The listing builds one solid part. Answer for the finished solid, in the listing's coordinates (mm). Face numbers are marked on the shaded views. Coordinates: 2 decimals unless noted, no trailing zeros. Write each loop counter-clockwise with the first axis right and the second up, starting at its lowest first coordinate (ties: lowest second). Pieces come first, ordered by that corner, then holes. Notation, with made-up numbers: M 6,21.25 L 47,21.25 A27 cw 47,52.25 Z; hole C -2,66.25 d8. An arc over 180 degrees is marked long. Answer as CSV lines item,"result". Start each with the question number.
```python
from build123d import *

# Parameters (mm, degrees)
SKETCH1_W                            = 398.78
SKETCH1_H                            = 101.6
BOSS_EXTRUDE1_DEPTH                  = 3.81
SKETCH11_W                           = 100.33
SKETCH11_H                           = 25.4
CUT_EXTRUDE1_DEPTH                   = 206.794869227
F_5_16_0_3125_DIAMETER_HOLE1_D       = 7.9375
F_6_CLEARANCE_HOLE1_D                = 3.6576
F_8_CLEARANCE_HOLE1_D                = 4.4958
LPATTERN1_COUNT                      = 2
LPATTERN1_PITCH                      = 328.93
F_11_64_0_17188_DIAMETER_HOLE2_D     = 4.365752
F_11_64_0_17188_DIAMETER_HOLE2_DEPTH = 8.89
F_11_64_0_17188_DIAMETER_HOLE2_TIP   = 1.311604225


with BuildPart() as part:
    # Sketch1 → Boss-Extrude1 (new body)
    with BuildSketch(Plane.XY):
        Rectangle(SKETCH1_W, SKETCH1_H)
    extrude(amount=BOSS_EXTRUDE1_DEPTH)

    # Sketch11 → Cut-Extrude1 (cut, through all)
    with BuildSketch(Plane.XY.offset(3.81)):
        with Locations((-53.975, -38.1)):
            Rectangle(SKETCH11_W, SKETCH11_H)
    extrude(amount=-CUT_EXTRUDE1_DEPTH, mode=Mode.SUBTRACT)

    # 5/16 (0.3125) Diameter Hole1 (through all)
    with Locations(Plane.XY.offset(3.81)):
        with Locations((11.074908, -43.18)):
            Hole(F_5_16_0_3125_DIAMETER_HOLE1_D / 2)

    # #6 Clearance Hole1 (through all)
    with Locations(Plane.XY.offset(3.81)):
        with Locations((132.715, -15.24), (196.215, -16.51), (196.215, 12.7), (196.215, 38.1), (132.715, 45.72), (132.715, 15.24), (132.715, -45.72), (196.215, -45.72)):
            f_6_clearance_hole1 = Hole(F_6_CLEARANCE_HOLE1_D / 2)

    # #8 Clearance Hole1 (through all)
    with Locations(Plane.XY.offset(3.81)):
        with Locations((180.34, 44.45), (180.34, 19.05), (180.34, -6.35), (-116.84, 44.45), (-116.84, 19.05), (-116.84, -6.35)):
            Hole(F_8_CLEARANCE_HOLE1_D / 2)

    # LPattern1: #6 Clearance Hole1 ×2
    with Locations(*[(-i * LPATTERN1_PITCH, 0, 0) for i in range(1, LPATTERN1_COUNT)]):
        add(f_6_clearance_hole1, mode=Mode.SUBTRACT)

    # 11/64 (0.17188) Diameter Hole2
    with Locations(Plane.XY.offset(3.81)):
        with Locations((-5.715, 6.35), (6.985, 6.35)):
            Hole(F_11_64_0_17188_DIAMETER_HOLE2_D / 2, depth=F_11_64_0_17188_DIAMETER_HOLE2_DEPTH)
            with Locations((0, 0, -(F_11_64_0_17188_DIAMETER_HOLE2_DEPTH + F_11_64_0_17188_DIAMETER_HOLE2_TIP / 2))):  # 118° drill point
                Cone(0, F_11_64_0_17188_DIAMETER_HOLE2_D / 2, F_11_64_0_17188_DIAMETER_HOLE2_TIP, mode=Mode.SUBTRACT)


solid = part.part
```
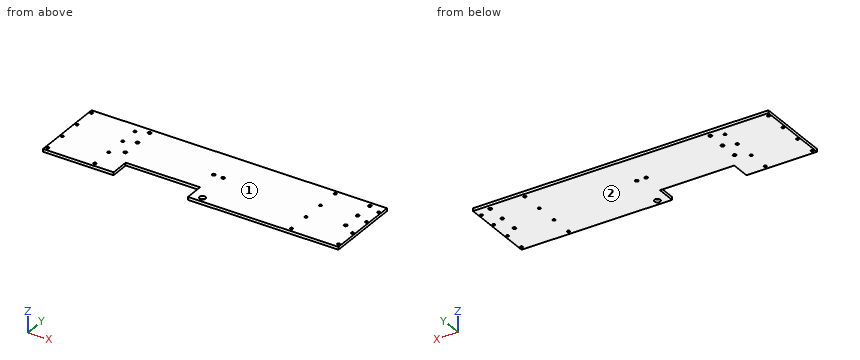
1) The part is cut by section C-C (x = -49). Determine the outline of the cut face in (y, z), then the cut area to 3 significant figures.
2) For a pull along Z with two mould halves and no side action, classify the marked faces 1 and 2 as +Z half, -Z half, draft (parallel to the pull), parting line (faces both ways), or undercut.
3) The part is cut by section A-A (y = -30). Determine the outline of the cut face in (x, z).
4) This flat-tipped pin is pushed along its axis until it touches: P1, Ø2, axis at x = 196.215, y = 12.7, coming from the -Z side. Where does it stop, or does it pass through?
5) Find the intervals of material crossed by line 1 (X direction, y = 18.5, z = 1.25); line 2 (X direction, y = -26, z = 3.3); line 3 (X direction, y = 14, z = 3.45), in increasing order. Write a range as from..to.
6) The part is cut by section B-B (z = 1.8). Count the separate pieces of the cut face and the enclosed holes in it, then the cut area to 3 significant figures.
Completed:
1,outline,"M -25.4,0 L 50.8,0 L 50.8,3.81 L -25.4,3.81 Z"
1,area,"290 mm²"
2,face 1,"+Z half"
2,face 2,"-Z half"
3,outline,"M -199.39,0 L -104.14,0 L -104.14,3.81 L -199.39,3.81 Z; M -3.81,0 L 199.39,0 L 199.39,3.81 L -3.81,3.81 Z"
4,P1,"through"
5,line 1,"-199.39..-119.02, -114.66..178.16, 182.52..199.39"
5,line 2,"-199.39..-104.14, -3.81..199.39"
5,line 3,"-199.39..-197.56, -194.87..-134, -131.43..131.37, 134.06..194.93, 197.5..199.39"
6,separate pieces,"1"
6,enclosed holes,"25"
6,area,"37,600 mm²"
